```python
from build123d import *

# Parameters (mm, degrees)
SKETCH1_W                  = 7.4
SKETCH1_H                  = 2.4
BOSS_EXTRUDE1_DEPTH        = 1.2
HOLE1_D                    = 0.6
HOLE1_DEPTH                = 1.2
HOLE1_CBORE_D              = 1
HOLE1_CBORE_DEPTH          = 0.9
HOLE1_TIP                  = 0.180258186
SKETCH11_W                 = 9.4
SKETCH11_H                 = 1.5
BOSS_EXTRUDE5_DEPTH        = 2
FILLET1_R                  = 2
F_0_8_0_8_DIAMETER_HOLE1_D = 0.8
M1_0_CLEARANCE_HOLE1_D     = 1.2


with BuildPart() as part:
    # Sketch1 → Boss-Extrude1 (new body)
    with BuildSketch(Plane.XY.offset(1.2)):
        with Locations((3.7, 1.2)):
            Rectangle(SKETCH1_W, SKETCH1_H)
        Polygon((8.4, 0), (7.4, 0), (0, 0), (-1, 0), (-1, -1.5), (8.4, -1.5), align=None)
    extrude(amount=-BOSS_EXTRUDE1_DEPTH)

    # Hole1
    with Locations(Plane.XY.offset(1.2)):
        with Locations((6.2, 1.2), (1.2, 1.2)):
            CounterBoreHole(HOLE1_D / 2, HOLE1_CBORE_D / 2, HOLE1_CBORE_DEPTH, depth=HOLE1_DEPTH)
            with Locations((0, 0, -(HOLE1_DEPTH + HOLE1_TIP / 2))):  # 118° drill point
                Cone(0, HOLE1_D / 2, HOLE1_TIP, mode=Mode.SUBTRACT)

    # Sketch11 → Boss-Extrude5 (add)
    with BuildSketch(Plane(origin=(0, 0, 0), x_dir=(-1, 0, 0), z_dir=(0, 0, -1))):
        with Locations((-3.7, -0.75)):
            Rectangle(SKETCH11_W, SKETCH11_H)
    extrude(amount=BOSS_EXTRUDE5_DEPTH)

    # Fillet1
    # the kernel refuses this fillet: 2 mm, written as the material it adds along each edge
    with BuildSketch(Plane(origin=(0, 0, 1.2), x_dir=(-1, 0, 0), z_dir=(0, 0, -1))) as fillet1_piece_1:
        with BuildLine():
            CenterArc((2, 1.732050808), FILLET1_R, 180, 60)
            Line((0, 1.732050808), (-0.04, 1.732050808))
            Line((-0.04, 1.732050808), (-0.04, 0))
            Line((-0.04, 0), (0, -0.04))
            ThreePointArc((0, -0.04), (0.5, -0.04), (0.98, -0.034641016))
            Line((0.98, -0.034641016), (1, 0))
        make_face()
    extrude(amount=1.2)
    with BuildSketch(Plane(origin=(7.4, 0, 1.2), x_dir=(1, 0, 0), z_dir=(0, 0, -1))) as fillet1_piece_2:
        with BuildLine():
            CenterArc((2, -1.732050808), FILLET1_R, 120, 60)
            Line((0, -1.732050808), (-0.04, -1.732050808))
            Line((-0.04, -1.732050808), (-0.04, 0))
            Line((-0.04, 0), (0, 0.04))
            ThreePointArc((0, 0.04), (0.5, 0.04), (0.98, 0.034641016))
            Line((0.98, 0.034641016), (1, 0))
        make_face()
    extrude(amount=1.2)

    # Ø0.8 (0.8) Diameter Hole1 (through all)
    with Locations(Plane.XY.offset(1.2)):
        with Locations((-0.2, -0.9), (7.6, -0.9)):
            Hole(F_0_8_0_8_DIAMETER_HOLE1_D / 2)

    # M1.0 Clearance Hole1 (through all)
    with Locations(Plane.XY.offset(1.2)):
        with Locations((3.7, 1.2)):
            Hole(M1_0_CLEARANCE_HOLE1_D / 2)


solid = part.part
```
Build history of the part. All positions in model axes, mm. A direction names the side the tool comes from. Round coordinates to 2 decimals unless told otherwise and drop trailing zeros. Write each loop counter-clockwise with the first axis right and the second up, starting at its lowest first coordinate (ties: lowest second). Pieces come first, ordered by that corner, then holes. Notation, with made-up numbers: (-25, 78) - (24, 78) arc R12 cw to (24, 86) - close; hole circle Ø10 at (41, -32). An arc over 180 degrees is marked (long way). Write each question's results on one line, items separated by ' | '. Start each with the question number.
Item 1: Saw through at A-A (y = -0.9). Write the cut outline in (x, z).
Item 2: Which spindle directions (+Z, -Z, +X, -X, +Y, -Y) get a long thin tool onto all of the face, cutting with end or side? Do faces 4 (the face through (4, -1, -2)), 5 (the face through (5.7, 1.2, 0.8)), 6 (the face through (3.8, 0.4, 0)). Say none if no direction does.
Item 3: Wall check: L1, parallel to Y at x = 6.2, z = 0.15; L2, parallel to Y at x = 6.2, z = 0.8; L3, parallel to X at y = -0.95, z = -0.8. Give the ranges that are in metal, low to high. Write a range as [from, to].
Item 4: Saw through at C-C (z = -0.75). Write the cut outline in (x, y), and give its area (3 significant figures).
Item 5: Saw through at D-D (y = 1.2). Write the cut outline in (x, z).
Item 6: Mould opens along X. For faces 1 (the face through (1.431, 0.756, 0.756)), 2 (the face through (7.675, 0.719, 0.608)), 3 (the face through (4, 0, -1)) say: pulls with the +X half, pulls with the -X half, needs draft (parallel to the pull), parting line crosses it, or undercut.
Item 7: Saw through at B-B (x = -0.2). Write the cut outline in (y, z).
Item 8: Drop flat-ended pins along their axis: P1, Ø1, axis at x = 2, z = -1.5, coming from the +Y side; P2, Ø1.2, axis at x = 4, y = 1, coming from the -Z side; P3, Ø0.5, axis at y = 2, z = 0.5, coming from the -X side. Give the stop position or say it passes through.
Results are:
1) outline: (-1, -2) - (-0.6, -2) - (-0.6, 1.2) - (-1, 1.2) - close; (0.2, -2) - (7.2, -2) - (7.2, 1.2) - (0.2, 1.2) - close; (8, -2) - (8.4, -2) - (8.4, 1.2) - (8, 1.2) - close
2) face 4: -Z, +X, -X, +Y, -Y | face 5: +Z | face 6: -Z, +X, -X, +Y
3) L1: y = [-1.5, 0.9], [1.5, 2.4] | L2: y = [-1.5, 0.7], [1.7, 2.4] | L3: x = [-1, -0.6], [0.2, 7.2], [8, 8.4]
4) outline: (-1, -1.5) - (8.4, -1.5) - (8.4, 0) - (-1, 0) - close; hole circle Ø0.8 at (-0.2, -0.9); hole circle Ø0.8 at (7.6, -0.9) | area: 13.1 mm²
5) outline: (-0.07, 0) - (0.9, 0) - (0.9, 0.3) - (0.7, 0.3) - (0.7, 1.2) - (-0.07, 1.2) - close; (1.5, 0) - (3.1, 0) - (3.1, 1.2) - (1.7, 1.2) - (1.7, 0.3) - (1.5, 0.3) - close; (4.3, 0) - (5.9, 0) - (5.9, 0.3) - (5.7, 0.3) - (5.7, 1.2) - (4.3, 1.2) - close; (6.5, 0) - (7.47, 0) - (7.47, 1.2) - (6.7, 1.2) - (6.7, 0.3) - (6.5, 0.3) - close
6) face 1: undercut | face 2: pulls with the +X half | face 3: needs draft
7) outline: (-1.5, -2) - (-1.3, -2) - (-1.3, 1.2) - (-1.5, 1.2) - close; (-0.5, -2) - (0, -2) - (0, 0) - (0.86, 0) - (0.86, 1.2) - (-0.5, 1.2) - close
8) P1: stops at y = 0 | P2: stops at z = 0 | P3: stops at x = 0
